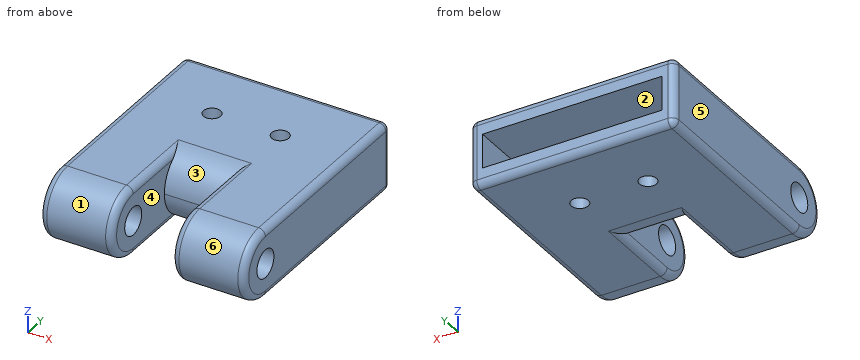
```python
from build123d import *

# Parameters (mm, degrees)
ESQUISSE1_W             = 38.1
ESQUISSE1_H             = 12.7
BOSS_EXTRU_1_DEPTH      = 3.175
ESQUISSE2_W             = 38.1
ESQUISSE2_H             = 12.7
ESQUISSE2_W_2           = 33.4518
ESQUISSE2_H_2           = 6.35
BOSS_EXTRU_2_DEPTH      = 25.4
ESQUISSE3_R             = 1.6
ENL_V_MAT_EXTRU_1_DEPTH = 25.4
ESQUISSE4_R             = 2.6
BOSS_EXTRU_3_DEPTH      = 13.49375
CONG_1_R                = 6.35
CONG_2_R                = 1.27


with BuildPart() as part:
    # Esquisse1 → Boss.-Extru.1 (new body)
    with BuildSketch(Plane(origin=(0, 0, 0), x_dir=(1, 0, 0), z_dir=(0, 1, 0))):
        Rectangle(ESQUISSE1_W, ESQUISSE1_H)
    extrude(amount=BOSS_EXTRU_1_DEPTH)

    # Esquisse2 → Boss.-Extru.2 (add)
    with BuildSketch(Plane(origin=(0, 3.175, 0), x_dir=(1, 0, 0), z_dir=(0, 1, 0))):
        Rectangle(ESQUISSE2_W, ESQUISSE2_H)
        Rectangle(ESQUISSE2_W_2, ESQUISSE2_H_2, mode=Mode.SUBTRACT)
    extrude(amount=BOSS_EXTRU_2_DEPTH)

    # Esquisse3 → Enlèv. mat.-Extru.1 (cut)
    with BuildSketch(Plane.XY.offset(6.35)):
        with Locations((-6.35, 15.875)):
            Circle(ESQUISSE3_R)
        with Locations((6.35, 15.875)):
            Circle(ESQUISSE3_R)
    extrude(amount=-ENL_V_MAT_EXTRU_1_DEPTH, mode=Mode.SUBTRACT)

    # Esquisse4 → Boss.-Extru.3 (add)
    with BuildSketch(Plane(origin=(19.05, 0, 0), x_dir=(0, 0, -1), z_dir=(1, 0, 0))):
        with BuildLine():
            Line((-6.35, 0), (-6.35, -9.525))
            ThreePointArc((-6.35, -9.525), (0, -15.875), (6.35, -9.525))
            Line((6.35, -9.525), (6.35, 0))
            Line((6.35, 0), (-6.35, 0))
        make_face()
        with Locations((0, -9.525)):
            Circle(ESQUISSE4_R, mode=Mode.SUBTRACT)
    boss_extru_3 = extrude(amount=-BOSS_EXTRU_3_DEPTH)

    # Symétrie1: Boss.-Extru.3 across plane
    add(boss_extru_3.mirror(Plane(origin=(0, 0, 0), x_dir=(0, 0, 1), z_dir=(1, 0, 0))))

    # Congé1
    cong_1_edges = [part.edges().sort_by_distance(p)[0] for p in [
        (0, 0, -6.35),
        (0, 0, 6.35),
    ]]
    fillet(cong_1_edges, radius=CONG_1_R - 0.0001)  # a hair under: the kernel refuses the full size

    # Congé2
    cong_2_edges = [part.edges().sort_by_distance(p)[0] for p in [
        (-19.05, 28.575, 0),
        (0, 28.575, 6.35),
        (19.05, 28.575, 0),
        (0, 28.575, -6.35),
        (5.55625, -1.58755, -6.35),
        (5.55625, -15.875, 0),
        (5.55625, -1.58755, 6.35),
        (19.05, -15.875, 0),
        (-5.55625, -1.58755, 6.35),
        (-5.55625, -15.875, 0),
        (-5.55625, -1.58755, -6.35),
        (-19.05, -15.875, 0),
        (19.05, 9.525, 6.35),
        (-19.05, 9.525, 6.35),
        (-19.05, 9.525, -6.35),
        (19.05, 9.525, -6.35),
    ]]
    fillet(cong_2_edges, radius=CONG_2_R)


solid = part.part
```
Could you check a few things on this model? Use its own coordinates, in mm. Face numbers are marked on the shaded views. A direction names the side the tool comes from. Coordinates: 2 decimals unless noted, no trailing zeros. Write each loop counter-clockwise with the first axis right and the second up, starting at its lowest first coordinate (ties: lowest second). Pieces come first, ordered by that corner, then holes. Notation, with made-up numbers: (76.25, 40) -> (107.25, 40) arc R23 cw to (107.25, 55) -> close; hole circle Ø10 at (-5, -27). An arc over 180 degrees is marked (long way). Write item = value, one per line. Start each with the question number.
(1) I want a section at A-A (y = -5.5). Please give me the cut outline in (x, z), plus the area to 3 significant figures.
(2) Which directions (+Z, -Z, +X, -X, +Y, -Y) give clear straight access to the entire face, cutting with the end or side of a thin tool? Please do the marked faces 1, 2 and 3.
(3) I need wall thicknesses on line 1 (Z direction, x = -15.5, y = 9.5) (3 decimals); line 2 (Y direction, x = 15.75, z = 0) (3 decimals); line 3 (X direction, y = -7, z = 4.5). Which ranges of each line are inside material? Lowest first, please. Write a range as [from, to].
(4) I want a section at B-B (y = 24.5). Please give me the cut outline in (x, z) (3 decimals).
(5) I want a section at D-D (z = 0.5). Give the number of separate pieces and of enclosed holes in the cut face, plus the area to 3 significant figures.
(6) Will these pins go through, and if not, where does the flat tip stop? pin 1 (1 mm diameter, centred on x = 12.5, z = 1.5, fed in from -Y); pin 2 (4 mm diameter, centred on x = -6.35, y = 15.875, fed in from -Z); pin 3 (3 mm diameter, centred on x = -4, z = 1, fed in from +Y) (3 decimals); pin 4 (1 mm diameter, centred on x = -4, z = 4.5, fed in from -Y).
(7) I want a section at C-C (x = -8.5). Please give me the cut outline in (y, z) (3 decimals), plus the area to 3 significant figures.
(8) We'd pull the mould along X, two halves only. Please class the marked faces 4, 5 and 6: released by +X, released by -X, zero draft, split by the parting line, or undercut.
Result set:
q1.outline = (-19.05, -5.08) arc R1.27 ccw to (-17.78, -6.35) -> (-6.83, -6.35) arc R1.27 ccw to (-5.56, -5.08) -> (-5.56, 5.08) arc R1.27 ccw to (-6.83, 6.35) -> (-17.78, 6.35) arc R1.27 ccw to (-19.05, 5.08) -> close; (5.56, -5.08) arc R1.27 ccw to (6.83, -6.35) -> (17.78, -6.35) arc R1.27 ccw to (19.05, -5.08) -> (19.05, 5.08) arc R1.27 ccw to (17.78, 6.35) -> (6.83, 6.35) arc R1.27 ccw to (5.56, 5.08) -> close
q1.area = 340 mm2
q2.face_1 = +X, -X, -Y
q2.face_2 = +Y
q2.face_3 = +Z, -Y
q3.line_1 = [-6.35, -3.175], [3.175, 6.35]
q3.line_2 = [-15.875, -12.125], [-6.925, 3.175]
q3.line_3 = [-19.05, -5.56], [5.56, 19.05]
q4.outline = (-19.05, -5.08) arc R1.27 ccw to (-17.78, -6.35) -> (17.78, -6.35) arc R1.27 ccw to (19.05, -5.08) -> (19.05, 5.08) arc R1.27 ccw to (17.78, 6.35) -> (-17.78, 6.35) arc R1.27 ccw to (-19.05, 5.08) -> close; hole (-16.726, -3.175) -> (16.726, -3.175) -> (16.726, 3.175) -> (-16.726, 3.175) -> close
q5.separate_pieces = 3
q5.enclosed_holes = 0
q5.area = 527 mm2
q6.pin_1 = -15.8
q6.pin_2 = -6.35
q6.pin_3 = 3.175
q6.pin_4 = 1.42
q7.outline = (-9.525, -6.35) -> (27.305, -6.35) arc R1.27 ccw to (28.575, -5.08) -> (28.575, -3.175) -> (3.175, -3.175) -> (3.175, 3.175) -> (28.575, 3.175) -> (28.575, 5.08) arc R1.27 ccw to (27.305, 6.35) -> (-9.525, 6.35) arc R6.35 ccw to start; hole circle Ø5.2 at (-9.525, 0)
q7.area = 364 mm2
q8.face_4 = undercut
q8.face_5 = released by -X
q8.face_6 = zero draft
